```python
from build123d import *

# Parameters (mm, degrees)
SKETCH_1_R      = 3
SKETCH_1_R_2    = 1
SKETCH_1_W      = 17
SKETCH_1_H      = 12
EXTRUDE_1_DEPTH = 1
EXTRUDE_2_DEPTH = 1
EXTRUDE_3_DEPTH = 2
SKETCH_5_W      = 10.2
SKETCH_5_H      = 9
EXTRUDE_4_DEPTH = 2
SKETCH_5_3_W    = 4.2
SKETCH_5_3_H    = 8.3
EXTRUDE_5_DEPTH = 3.1
SHELL_1_T       = -0.5
SKETCH_6_W      = 0.2
SKETCH_6_H      = 0.2
EXTRUDE_6_DEPTH = 2
FILLET_1_R      = 0.2


with BuildPart() as part:
    # Sketch 1 → Extrude 1 (new body)
    # profile 1 of 5: a face of its own
    with BuildSketch(Plane(origin=(0, 0, 0), x_dir=(1, 0, 0), z_dir=(0, 1, 0))):
        with Locations((-5.5, 6)):
            Circle(SKETCH_1_R)
        with Locations(Location((-5.5, 7, 0), (0, 0, 270))):
            Circle(SKETCH_1_R_2, mode=Mode.SUBTRACT)
    # profile 2 of 5: a face of its own
    with BuildSketch(Plane(origin=(0, 0, 0), x_dir=(1, 0, 0), z_dir=(0, 1, 0))):
        with Locations((5.5, 6)):
            Circle(SKETCH_1_R)
        with Locations(Location((5.5, 7, 0), (0, 0, 270))):
            Circle(SKETCH_1_R_2, mode=Mode.SUBTRACT)
    # profile 3 of 5: a face of its own
    with BuildSketch(Plane(origin=(0, 0, 0), x_dir=(1, 0, 0), z_dir=(0, 1, 0))):
        with Locations((-5.5, -6)):
            Circle(SKETCH_1_R)
        with Locations(Location((-5.5, -7, 0), (0, 0, 270))):
            Circle(SKETCH_1_R_2, mode=Mode.SUBTRACT)
    # profile 4 of 5: a face of its own
    with BuildSketch(Plane(origin=(0, 0, 0), x_dir=(1, 0, 0), z_dir=(0, 1, 0))):
        with Locations((5.5, -6)):
            Circle(SKETCH_1_R)
        with Locations(Location((5.5, -7, 0), (0, 0, 270))):
            Circle(SKETCH_1_R_2, mode=Mode.SUBTRACT)
    # profile 5 of 5: a face of its own
    with BuildSketch(Plane(origin=(0, 0, 0), x_dir=(1, 0, 0), z_dir=(0, 1, 0))):
        Rectangle(SKETCH_1_W, SKETCH_1_H)
    extrude(amount=EXTRUDE_1_DEPTH)

    # Sketch 3 → Extrude 2 (add)
    with BuildSketch(Plane(origin=(0, 1, 0), x_dir=(1, 0, 0), z_dir=(0, 1, 0))):
        with BuildLine():
            Line((-2.3, -3.5), (2.3, -3.5))
            ThreePointArc((2.3, -3.5), (5.8, 0), (2.3, 3.5))
            Line((2.3, 3.5), (-2.3, 3.5))
            ThreePointArc((-2.3, 3.5), (-5.8, 0), (-2.3, -3.5))
        make_face()
        with BuildLine():
            ThreePointArc((2.3, -2.5), (4.8, 0), (2.3, 2.5))
            Line((2.3, 2.5), (-2.3, 2.5))
            ThreePointArc((-2.3, 2.5), (-4.8, 0), (-2.3, -2.5))
            Line((-2.3, -2.5), (2.3, -2.5))
        make_face(mode=Mode.SUBTRACT)
    extrude(amount=EXTRUDE_2_DEPTH)

    # Sketch 3_3 → Extrude 3 (add)
    with BuildSketch(Plane(origin=(0, 1, 0), x_dir=(1, 0, 0), z_dir=(0, 1, 0))):
        with BuildLine():
            Line((-2.3, 2.5), (2.3, 2.5))
            ThreePointArc((2.3, 2.5), (4.8, 0), (2.3, -2.5))
            Line((2.3, -2.5), (-2.3, -2.5))
            ThreePointArc((-2.3, -2.5), (-4.8, 0), (-2.3, 2.5))
        make_face()
    extrude(amount=EXTRUDE_3_DEPTH)

    # Sketch 5 → Extrude 4 (add)
    with BuildSketch(Plane.XZ):
        with Locations((2.2, 0)):
            Rectangle(SKETCH_5_W, SKETCH_5_H)
    extrude(amount=EXTRUDE_4_DEPTH)



with BuildPart() as body_2:
    # Sketch 5_3 → Extrude 5 (new body)
    with BuildSketch(Plane.XZ):
        with Locations((-6.4, 0)):
            Rectangle(SKETCH_5_3_W, SKETCH_5_3_H)
    extrude(amount=EXTRUDE_5_DEPTH)

    # Shell 1
    shell_1_openings = [body_2.faces().sort_by_distance(p)[0] for p in [
        (-8.5, -1.55, 0),
    ]]
    offset(amount=SHELL_1_T, openings=shell_1_openings, kind=Kind.INTERSECTION)


with BuildPart() as part_1:
    add(part.part)

    add(body_2.part)  # Extrude 6 merges body 2
    # Sketch 6 → Extrude 6 (add)
    with BuildSketch(Plane.ZY.offset(4.8)):
        with Locations((1.5, -2)):
            Rectangle(SKETCH_6_W, SKETCH_6_H)
        with Locations((2.5, -2)):
            Rectangle(SKETCH_6_W, SKETCH_6_H)
        with Locations((0.5, -2)):
            Rectangle(SKETCH_6_W, SKETCH_6_H)
        with Locations((-0.5, -2)):
            Rectangle(SKETCH_6_W, SKETCH_6_H)
        with Locations((-1.5, -2)):
            Rectangle(SKETCH_6_W, SKETCH_6_H)
        with Locations((-2.5, -2)):
            Rectangle(SKETCH_6_W, SKETCH_6_H)
    extrude(amount=EXTRUDE_6_DEPTH)

    # Fillet 1
    fillet_1_edges = [part_1.edges().sort_by_distance(p)[0] for p in [
        (7.3, -2, 0),
        (7.3, -1, -4.5),
        (2.2, -2, 4.5),
        (7.3, -1, 4.5),
        (-2.9, -1, 4.5),
        (-2.9, -1, -4.5),
        (-2.9, -2, 0),
        (2.2, -2, -4.5),
    ]]
    fillet(fillet_1_edges, radius=FILLET_1_R)


solid = part_1.part
```
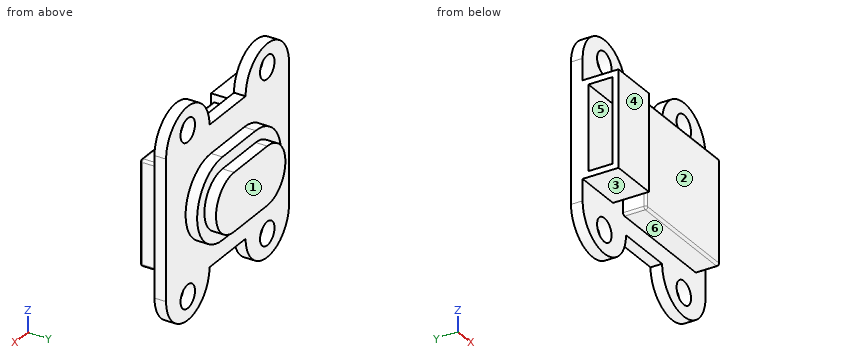
Model file for the job. Use its own axes, mm. Face numbers are marked on the shaded views. A direction names the side the tool comes from. Coordinates: 2 decimals unless noted, no trailing zeros. Loops run counter-clockwise (first coordinate to the right, second up) from the corner with the lowest first, then second, coordinate; pieces in that order, holes last. Notation, with made-up numbers: (66, 72) - (106, 72) arc R14 ccw to (106, 84) - close; hole circle Ø3 at (9, -26). An arc over 180 degrees is marked (long way). Answer as a JSON object with one key per item and string values. Group by question number.
(1) Cut at D-D (z = -7). Give the cut face in (x, y).
(2) Cut at B-B (x = 0.5). Give the cut face in (y, z), then the cut area to 3 significant figures.
(3) Cut at A-A (y = -1.5). Give the cut face in (x, z).
(4) Cut at C-C (y = 0.25). Give the cut face in (x, z).
(5) Flat gauge pins, fed straight in: pin 1 (0.5 mm diameter, centred on x = -1, y = 0.5, fed in from -Z); pin 2 (5 mm diameter, centred on x = -1.5, z = -0.5, fed in from -Y); pin 3 (2.5 mm diameter, centred on x = 5.5, z = -7, fed in from +Y). Where does each tip first touch, or does it go through?
(6) Two-plate mould, pull along Y, no slides. Class the marked faces 4, 5 and 6: released by +Y, released by -Y, zero draft, split by the parting line, or undercut.
(7) Probe line 1 along X through (y, z) = (0.55, -7); line 2 along Y through (x, z) = (-6, -3); line 3 along Y through (x, z) = (7.5, 6.25). List the from-to ranges inside material, lowest first.
(8) Tool access for the marked faces 1, 2 and 3: list every direction of +Z, -Z, +X, -X, +Y, -Y with a clear straight run to the whole face (end or side of a thin tool).
Geometry says:
{
 "1": {"outline": "(-8.33, 0) - (-6.5, 0) - (-6.5, 1) - (-8.33, 1) - close; (-4.5, 0) - (-2.67, 0) - (-2.67, 1) - (-4.5, 1) - close; (2.67, 0) - (4.5, 0) - (4.5, 1) - (2.67, 1) - close; (6.5, 0) - (8.33, 0) - (8.33, 1) - (6.5, 1) - close"},
 "2": {"outline": "(-2, -4.3) arc R0.2 ccw to (-1.8, -4.5) - (0, -4.5) - (0, -6) - (1, -6) - (1, -3.5) - (2, -3.5) - (2, -2.5) - (3, -2.5) - (3, 2.5) - (2, 2.5) - (2, 3.5) - (1, 3.5) - (1, 6) - (0, 6) - (0, 4.5) - (-1.8, 4.5) arc R0.2 ccw to (-2, 4.3) - close", "area": "42.0 mm^2"},
 "3": {"outline": "(-8.5, -4.15) - (-4.3, -4.15) - (-4.3, 4.15) - (-8.5, 4.15) - (-8.5, 3.65) - (-4.8, 3.65) - (-4.8, -3.65) - (-8.5, -3.65) - close; (-2.9, -4.3) arc R0.2 ccw to (-2.7, -4.5) - (7.1, -4.5) arc R0.2 ccw to (7.3, -4.3) - (7.3, 4.3) arc R0.2 ccw to (7.1, 4.5) - (-2.7, 4.5) arc R0.2 ccw to (-2.9, 4.3) - close"},
 "4": {"outline": "(-8.5, -6) arc R3 ccw to (-2.5, -6) - (2.5, -6) arc R3 ccw to (8.5, -6) - (8.5, 6) arc R3 ccw to (2.5, 6) - (-2.5, 6) arc R3 ccw to (-8.5, 6) - close; hole circle Ø2 at (-5.5, -7); hole circle Ø2 at (-5.5, 7); hole circle Ø2 at (5.5, -7); hole circle Ø2 at (5.5, 7)"},
 "5": {"pin 1": "stops at z = -6", "pin 2": "stops at y = -2", "pin 3": "stops at y = 1"},
 "6": {"face 4": "released by -Y", "face 5": "undercut", "face 6": "zero draft"},
 "7": {"line 1": "x = -8.33 to -6.5, -4.5 to -2.67, 2.67 to 4.5, 6.5 to 8.33", "line 2": "y = -3.1 to -2.6, -0.5 to 1", "line 3": "y = 0 to 1"},
 "8": {"face 1": "+Z, -Z, +X, -X, +Y", "face 2": "+Z, -Z, +X, -Y", "face 3": "-Z, -X, -Y"}
}
